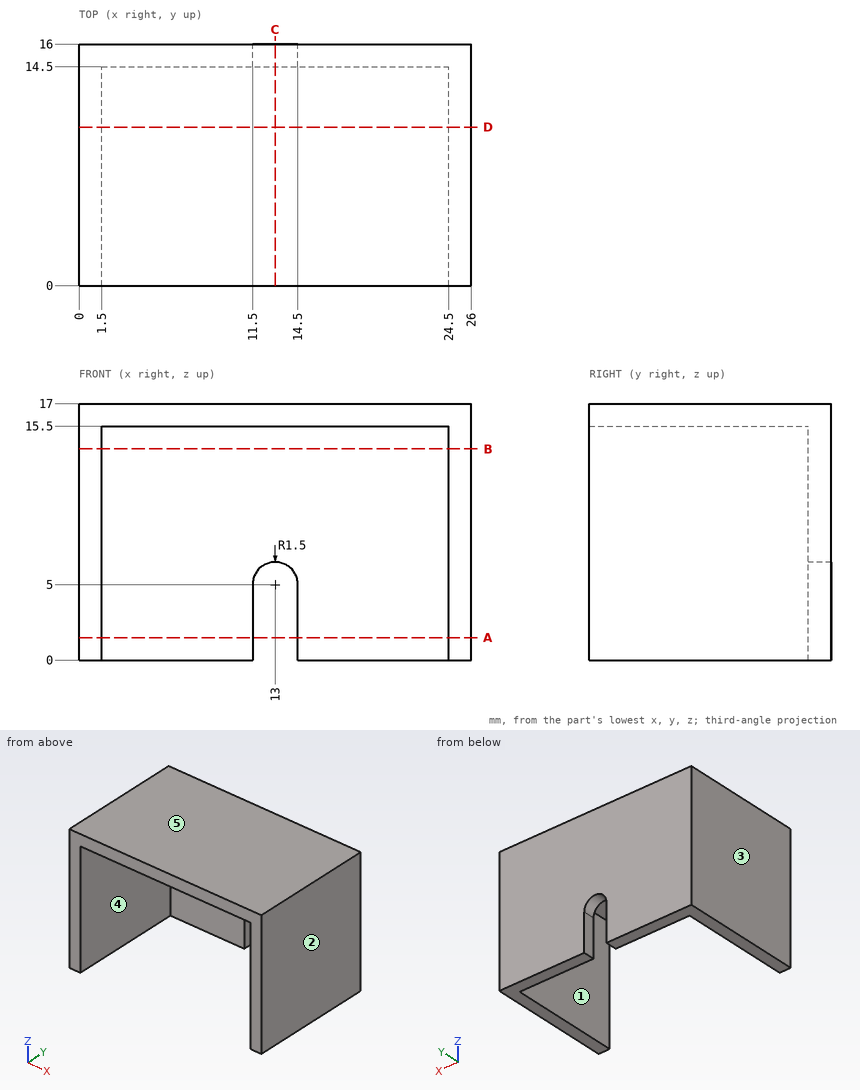
Design review of the part shown in the three views and the two pictorial views. Dimensions are in mm from the part's minimum x, y and z. A direction names the side the tool comes from. Give positions to 0.01 mm unless a question says otherwise; leave off trailing zeros. Loops run counter-clockwise (first coordinate to the right, second up) from the corner with the lowest first, then second, coordinate; pieces in that order, holes last. Notation, with made-up numbers: (12.5, -7.5) -> (52.5, -7.5) arc R28 ccw to (52.5, 27.5) -> close; hole circle Ø8 at (34.5, 7.5). An arc over 180 degrees is marked (long way). One line per item, written item: value.
Q1. Draft analysis for pull direction X (two halves, no side actions). For the marked faces 3, 4 and 5, state which applies: pulls with the +X half, pulls with the -X half, needs draft (parallel to the pull), parting line crosses it, or undercut.
Numbers:
face 3: pulls with the -X half
face 4: undercut
face 5: needs draft
Q2. We need section B-B on z = 14. Give the boundary of the cut face in (x, y).
Numbers:
outline: (0, 0) -> (1.5, 0) -> (1.5, 14.5) -> (24.5, 14.5) -> (24.5, 0) -> (26, 0) -> (26, 16) -> (0, 16) -> close
Q3. We need section A-A on z = 1.5. Give the boundary of the cut face in (x, y).
Numbers:
outline: (0, 0) -> (1.5, 0) -> (1.5, 14.5) -> (11.5, 14.5) -> (11.5, 16) -> (0, 16) -> close; (14.5, 14.5) -> (24.5, 14.5) -> (24.5, 0) -> (26, 0) -> (26, 16) -> (14.5, 16) -> close
Q4. For L1, parallel to X at y = 10, z = 3.25; L2, parallel to Y at x = 11.5, z = 10; L3, parallel to Z at x = 8.25, y = 3, list the stretches that pass through material, from the lowest coordinate up.
Numbers:
L1: x = 0 to 1.5, 24.5 to 26
L2: y = 14.5 to 16
L3: z = 15.5 to 17
Q5. We need section D-D on y = 10.5. Give the boundary of the cut face in (x, z).
Numbers:
outline: (0, 0) -> (1.5, 0) -> (1.5, 15.5) -> (24.5, 15.5) -> (24.5, 0) -> (26, 0) -> (26, 17) -> (0, 17) -> close
Q6. Machinability: for the marked faces 1 and 2, which of the approach directions +Z, -Z, +X, -X, +Y, -Y give a long, thin tool a straight path to every point of the face, cutting with its end or side? Answer none if there is none.
Numbers:
face 1: -Z, -Y
face 2: +Z, -Z, +X, +Y, -Y
Q7. For pin 1 Ø8 at (x, y) = (8.5, 3.5) entering from -Z; pin 2 Ø2 at (x, z) = (19, 10.5) entering from -Y, all flat-tipped, find the tip position at first contact; note any pin that passes through.
Numbers:
pin 1: stops at z = 15.5
pin 2: stops at y = 14.5
Q8. We need section C-C on x = 13. Give the boundary of the cut face in (y, z), and give its area (3 significant figures).
Numbers:
outline: (0, 15.5) -> (14.5, 15.5) -> (14.5, 6.5) -> (16, 6.5) -> (16, 17) -> (0, 17) -> close
area: 37.5 mm^2
